Build history of the part. All positions in model axes, mm. A direction names the side the tool comes from. Give positions to 0.01 mm unless a question says otherwise; leave off trailing zeros. Loops run counter-clockwise (first coordinate to the right, second up) from the corner with the lowest first, then second, coordinate; pieces in that order, holes last. Notation, with made-up numbers: (42, 75.25) - (67, 75.25) arc R31 ccw to (67, 113.25) - close; hole circle Ø2 at (79, -27). An arc over 180 degrees is marked (long way). Return JSON: item names as keys, results as strings. Group by question number.
1) 3-axis set-ups, long thin cutter, end or side, ignore diameter. For faces 1 (the face through (-529.925, 93.67, -228.183)), 2 (the face through (-38, 215, -75)), 3 (the face through (157, 94, 0)), 4 (the face through (-112, 92, 75)), 5 (the face through (0, 94, -508)): which of +Z, -Z, +X, -X, +Y, -Y reach the whole face in a straight line?
2) Slice it at B-B (y = 210). List the corners of the cut face in (x, z), and give its area (3 significant figures).
3) Slice it at A-A (y = 42.5). List the corners of the cut face in (x, z).
4) Slice it at D-D (y = 171). List the corners of the cut face in (x, z).
5) Drill centre lines: probe 1 along X at (y, z) = (70.5, -235); probe 2 along X at (y, z) = (49, -231); probe 3 along Y at (x, z) = (91, -135). Where is each one in solid material? Low to high. Write a range as from..to.
6) Slice it at C-C (x = -459). List the corners of the cut face in (y, z), and give its area (3 significant figures).
7) Drop flat-ended pins along their axis: pin 1 (8 mm diameter, centred on y = 151.5, z = -310.5, fed in from +X); pin 2 (5 mm diameter, centred on x = -14.5, z = -293.5, fed in from +Y); pin 3 (1 mm diameter, centred on x = 133, y = 106.5, fed in from -Z). Give the stop position or say it passes through.
8) Mould opens along Z. For faces 6 (the face through (310, 44, -238)), 7 (the face through (-170.425, 116.61, -241.509)), 8 (the face through (-112, 94, -545)) say: released by +Z, released by -Z, zero draft, split by the parting line, or undercut.
```python
from build123d import *

# Parameters (mm, degrees)
BOSS_EXTRUDE1_DEPTH = 190
SKETCH2_R           = 170
BOSS_EXTRUDE2_DEPTH = 40
BOSS_EXTRUDE2_TAPER = 25
SKETCH3_W           = 75
SKETCH3_H           = 150
BOSS_EXTRUDE3_DEPTH = 50
SKETCH4_R           = 50
CUT_EXTRUDE1_DEPTH  = 795.244924441
CUT_EXTRUDE2_DEPTH  = 798.198218764


with BuildPart() as part:
    # Sketch1 → Boss-Extrude1 (new body)
    with BuildSketch(Plane(origin=(0, 0, 0), x_dir=(1, 0, 0), z_dir=(0, 1, 0))):
        with BuildLine():
            Line((0, 0), (0, -75))
            Line((0, -75), (-220, -75))
            ThreePointArc((-220, -75), (-530, 235), (-220, 545))
            Line((-220, 545), (0, 545))
            Line((0, 545), (0, 470))
            Line((0, 470), (310, 470))
            Line((310, 470), (310, 0))
            Line((310, 0), (0, 0))
        make_face()
    extrude(amount=BOSS_EXTRUDE1_DEPTH)

    # Sketch2 → Boss-Extrude2 (add)
    with BuildSketch(Plane(origin=(0, 190, 0), x_dir=(1, 0, 0), z_dir=(0, 1, 0))):
        with Locations((-220, 235)):
            Circle(SKETCH2_R)
    extrude(amount=BOSS_EXTRUDE2_DEPTH, taper=BOSS_EXTRUDE2_TAPER)

    # Sketch3 → Boss-Extrude3 (add)
    with BuildSketch(Plane(origin=(0, 190, 0), x_dir=(1, 0, 0), z_dir=(0, 1, 0))):
        with Locations((-37.5, 0)):
            Rectangle(SKETCH3_W, SKETCH3_H)
    extrude(amount=BOSS_EXTRUDE3_DEPTH)

    # Sketch4 → Cut-Extrude1 (cut, through all)
    with BuildSketch(Plane(origin=(0, 230, 0), x_dir=(1, 0, 0), z_dir=(0, 1, 0))):
        with Locations(Location((-220, 235, 0), (0, 0, 270))):
            Circle(SKETCH4_R)
    extrude(amount=-CUT_EXTRUDE1_DEPTH, mode=Mode.SUBTRACT)

    # Sketch5 → Cut-Extrude2 (cut, through all)
    with BuildSketch(Plane.XY):
        Polygon((310, 190), (136.794919243, 190), (310, 90), align=None)
    extrude(amount=-CUT_EXTRUDE2_DEPTH, mode=Mode.SUBTRACT)


solid = part.part
```
Results:
{
 "1": {"face 1": "-X, +Y, -Y", "face 2": "+X, +Y", "face 3": "+Z, +X, +Y, -Y", "face 4": "+Z, +X, -X, +Y, -Y", "face 5": "-Z, +X, +Y, -Y"},
 "2": {"outline": "circle Ø321.35 at (-220, -235); (-75, -75) - (0, -75) - (0, 75) - (-75, 75) - close; hole circle Ø100 at (-220, -235)", "area": "84,500 mm2"},
 "3": {"outline": "(-220, -545) - (0, -545) - (0, -470) - (310, -470) - (310, 0) - (0, 0) - (0, 75) - (-220, 75) arc R310 ccw to start; hole circle Ø100 at (-220, -235)"},
 "4": {"outline": "(-220, -545) - (0, -545) - (0, -470) - (169.7, -470) - (169.7, 0) - (0, 0) - (0, 75) - (-220, 75) arc R310 ccw to start; hole circle Ø100 at (-220, -235)"},
 "5": {"probe 1": "-530..-270, -170..310", "probe 2": "-529.97..-269.84, -170.16..310", "probe 3": "0..190"},
 "6": {"outline": "(0, -432.43) - (190, -432.43) - (190, -37.57) - (0, -37.57) - close", "area": "75,000 mm2"},
 "7": {"pin 1": "x = 210.41", "pin 2": "y = 190", "pin 3": "z = -470"},
 "8": {"face 6": "zero draft", "face 7": "undercut", "face 8": "released by -Z"}
}
